Can you work these out from the model? Positions are in its coordinate system, mm. Face numbers are marked on the shaded views. A direction names the side the tool comes from. Round coordinates to 2 decimals unless told otherwise and drop trailing zeros. Write each loop counter-clockwise with the first axis right and the second up, starting at its lowest first coordinate (ties: lowest second). Pieces come first, ordered by that corner, then holes. Notation, with made-up numbers: M 69.25,-40 L 79.25,-40 A11 ccw 79.25,-30 Z; hole C 67.25,-17 d5. An arc over 180 degrees is marked long. Answer in a Markdown table with one row per item. Add a question column.
(1) I'm going to push flat-ended pins straight in: pin 1 (4 mm diameter, centred on y = 22, z = 6.5, fed in from +X); pin 2 (4 mm diameter, centred on y = 21, z = 3, fed in from -X); pin 3 (1.5 mm diameter, centred on y = -24.5, z = 2.5, fed in from +X). Where does each tip first touch, or does it pass through?
(2) If we mould it in two halves opening along Y, with no side actions, what happens to the marked faces 3 and 4? For each: released by +Y, released by -Y, zero draft, split by the parting line, or undercut.
(3) If I drill on probe 1 along Y at (x, z) = (0, 12); probe 2 along Y at (x, z) = (0, 3.75); probe 3 along X at (y, z) = (14.5, 3.5), over which ranges is the centre line in solid material (lowest first)?
(4) Suppose I cut it at D-D, the plane y = 44.5. Write out the boundary of the cut face in (x, z), then the cut area to 3 significant figures.
(5) Suppose I cut it at B-B, the plane x = -11.5. Write out the boundary of the cut face in (y, z).
(6) Suppose I cut it at C-C, the plane z = 13.5. Write out the boundary of the cut face in (x, y), then the cut area to 3 significant figures.
(7) Suppose I cut it at A-A, the plane y = 0. Write out the boundary of the cut face in (x, z), then the cut area to 3 significant figures.
(8) For the marked faces 1 and 2, which set-ups out of +Z, -Z, +X, -X, +Y, -Y let a thin tool reach every point of the face, with its end or its side?
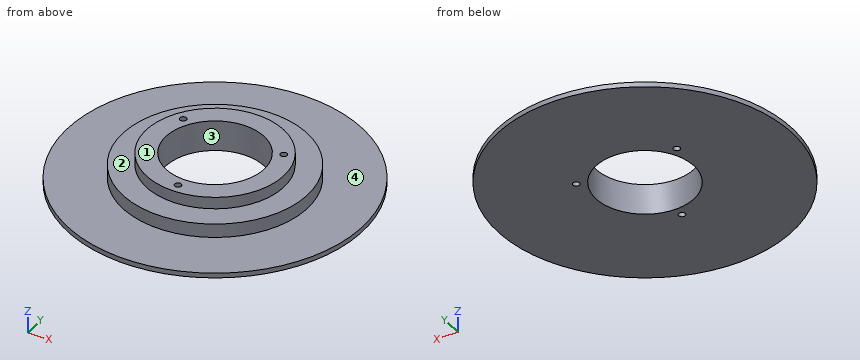
from build123d import *

# Parameters (mm, degrees)
SKETCH001_R   = 25
SKETCH001_R_2 = 1.7
POCKET_DEPTH  = 15.501


with BuildPart() as part:
    # Sketch → Revolution (revolve)
    with BuildSketch(Plane.XZ):
        Polygon((0, 15.5), (35, 15.5), (35, 9.5), (47, 9.5), (47, 2.5), (75, 2.5), (75, 0), (0, 0), align=None)
    revolve(axis=Axis((0, 0, 0), (0, 0, 1)))

    # Sketch001 → Pocket (cut, through all)
    with BuildSketch(Plane(origin=(0, 0, 15.5), x_dir=(-1, 0, 0), z_dir=(0, 0, 1))):
        Circle(SKETCH001_R)
        with Locations((0, 30)):
            Circle(SKETCH001_R_2)
        with Locations((25.980762, -15)):
            Circle(SKETCH001_R_2)
        with Locations((-25.980762, -15)):
            Circle(SKETCH001_R_2)
    extrude(amount=-POCKET_DEPTH, mode=Mode.SUBTRACT)


solid = part.part
Calculated:
| question | item | result |
|---|---|---|
| 1 | pin 1 | x = 42.53 |
| 1 | pin 2 | x = -72.54 |
| 1 | pin 3 | x = 71.14 |
| 2 | face 3 | undercut |
| 2 | face 4 | zero draft |
| 3 | probe 1 | -35 to -31.7, -28.3 to -25, 25 to 35 |
| 3 | probe 2 | -47 to -31.7, -28.3 to -25, 25 to 47 |
| 3 | probe 3 | -44.71 to -27.61, -24.36 to -20.37, 20.37 to 24.36, 27.61 to 44.71 |
| 4 | outline | M -60.37,0 L 60.37,0 L 60.37,2.5 L 15.12,2.5 L 15.12,9.5 L -15.12,9.5 L -15.12,2.5 L -60.37,2.5 Z |
| 4 | area | 514 mm² |
| 5 | outline | M -74.11,0 L -22.2,0 L -22.2,15.5 L -33.06,15.5 L -33.06,9.5 L -45.57,9.5 L -45.57,2.5 L -74.11,2.5 Z; M 22.2,0 L 74.11,0 L 74.11,2.5 L 45.57,2.5 L 45.57,9.5 L 33.06,9.5 L 33.06,15.5 L 22.2,15.5 Z |
| 6 | outline | C 0,0 d70; hole C -25.98,15 d3.4; hole C 0,0 d50; hole C 0,-30 d3.4; hole C 25.98,15 d3.4 |
| 6 | area | 1,860 mm² |
| 7 | outline | M -75,0 L -25,0 L -25,15.5 L -35,15.5 L -35,9.5 L -47,9.5 L -47,2.5 L -75,2.5 Z; M 25,0 L 75,0 L 75,2.5 L 47,2.5 L 47,9.5 L 35,9.5 L 35,15.5 L 25,15.5 Z |
| 7 | area | 678 mm² |
| 8 | face 1 | +Z, +X, -X, +Y, -Y |
| 8 | face 2 | +Z |
